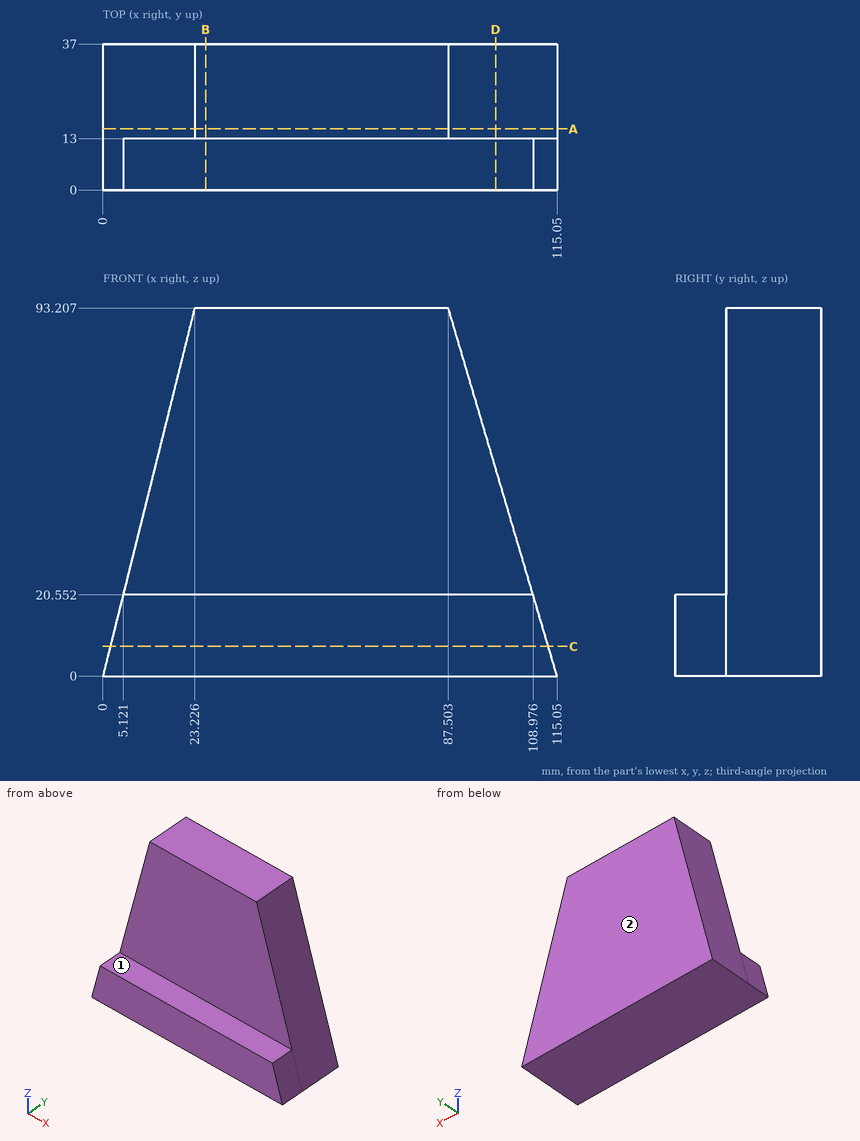
Answer from the drawing. Dimensions are ordinates in mm from the lowest x, y and z of the part. A direction names the side the tool comes from. Give positions to 0.01 mm unless a question says otherwise; leave off trailing zeros. Loops run counter-clockwise (first coordinate to the right, second up) from the corner with the lowest first, then second, coordinate; pieces in that order, holes last. Notation, with made-up numbers: (88, 51.5) -> (97, 51.5) arc R19 ccw to (97, 68.5) -> close; hole circle Ø1 at (-4.5, -37.5). An arc over 180 degrees is marked (long way). One line per question, with ' | ' between items. Start each with the question number.
1) For the marked faces 1 and 2, determine the directions among +Z, -Z, +X, -X, +Y, -Y from which every point of the face is accessible in a straight line to the end or side of a thin tool.
2) Section C-C, the plane z = 7.5 is taken. Determine the outline of the cut face in (x, y), then the cut area to 3 significant figures.
3) Section A-A, the plane y = 15.5 is taken. Determine the outline of the cut face in (x, z), then the cut area to 3 significant figures.
4) Straight lines are drawn through the part: L1, parallel to Y at x = 54, z = 50.5; L2, parallel to Z at x = 102, y = 4.5; L3, parallel to X at y = 20, z = 28 (1 decimal). For each, find the intervals that lie inside material, in ascending order.
5) Section D-D, the plane x = 99.5 is taken. Determine the outline of the cut face in (y, z).
6) Each of these flat-tipped pins is pushed along its axis until it touches: pin 1 (4 mm diameter, centred on x = 28, z = 32.5, fed in from -Y); pin 2 (10 mm diameter, centred on y = 11, z = 10, fed in from -X); pin 3 (3 mm diameter, centred on y = 30.5, z = 13.5, fed in from -X). Where does it stop, or does it pass through?
7) Section B-B, the plane x = 26 is taken. Determine the outline of the cut face in (y, z), then the cut area to 3 significant figures.
Resolved:
1) face 1: +Z, +X, -X, -Y | face 2: +Z, -Z, +X, -X, +Y
2) outline: (1.87, 0) -> (112.83, 0) -> (112.83, 37) -> (1.87, 37) -> close | area: 4,110 mm2
3) outline: (0, 0) -> (115.05, 0) -> (87.5, 93.21) -> (23.23, 93.21) -> close | area: 8,360 mm2
4) L1: 13 to 37 | L2: 0 to 20.55 | L3: 7 to 106.8
5) outline: (0, 0) -> (37, 0) -> (37, 52.61) -> (13, 52.61) -> (13, 20.55) -> (0, 20.55) -> close
6) pin 1: y = 13 | pin 2: x = 1.25 | pin 3: x = 2.99
7) outline: (0, 0) -> (37, 0) -> (37, 93.21) -> (13, 93.21) -> (13, 20.55) -> (0, 20.55) -> close | area: 2,500 mm2
